from build123d import *

# Parameters (mm, degrees)
F0_R     = 4
F0_W     = 4
F0_H     = 4
F1_DEPTH = 10
F2_W     = 4.25
F2_H     = 4.25
F3_DEPTH = 7
F4_DEPTH = 6


with BuildPart() as f1:
    # F0 (on Top) → F1 (new body)
    with BuildSketch(Plane.XY):
        Circle(F0_R)
        Rectangle(F0_W, F0_H, mode=Mode.SUBTRACT)
        Rectangle(F0_W, F0_H)
    extrude(amount=F1_DEPTH)

    # F2 (on face) → F3 (cut)
    with BuildSketch(Plane.XY.offset(10)):
        Rectangle(F2_W, F2_H)
    extrude(amount=-F3_DEPTH, mode=Mode.SUBTRACT)

    # F0 (on Top) → F4 (join)
    with BuildSketch(Plane.XY):
        Rectangle(F0_W, F0_H)
    extrude(amount=-F4_DEPTH)


solid = f1.part
The listing builds one solid part. Answer for the finished solid, in the listing's coordinates (mm). A direction names the side the tool comes from. Round coordinates to 2 decimals unless told otherwise and drop trailing zeros. Order: outer loops, then holes, each group sorted by start corner. A loop starts at its lowest first (then second) coordinate and runs counter-clockwise, first axis right, second up. Notation, with made-up numbers: M 38.5,4 L 47.5,4 A14 cw 47.5,22 Z; hole C -1,23 d2. An arc over 180 degrees is marked long. Answer in a Markdown table with one row per item. Add a question column.
1) Flat-ended cylindrical pins translate along their axes: pin 1 Ø1 at (x, y) = (0.5, -1) entering from +Z; pin 2 Ø3 at (x, z) = (-1, -3.5) entering from +Y; pin 3 Ø1 at (x, z) = (-2.5, 3.5) entering from +Y. Find the tip coordinate at first contact, or state that the pin passes through.
2) Which of the six approach directions +Z, -Z, +X, -X, +Y, -Y give full straight-line access (tool end or side, diameter ignored) to faces 4 (the face through (0, 0, -6)), 5 (the face through (0, -2, -3)), 6 (the face through (0, 2.125, 7)), 7 (the face through (-2, 0, -3)), 8 (the face through (0, 2, -3))?
3) Consider line 1 along Z through (x, y) = (-3.25, 2); line 2 along X through (y, z) = (1.5, -4); line 3 along X through (y, z) = (0.75, 4) (3 decimals). Determine where each line is inside the solid, lowest interval first. Write a range as from..to.
4) The part is cut by section C-C on z = 7. Determine the outline of the cut face in (x, y) (3 decimals).
5) Determine the mould class of faces 1 (the face through (-0.867, -3.905, 4.93)), 2 (the face through (2.125, 0, 7)), 3 (the face through (2, 0, -3)) for opening direction Y: pulls with the +Y half, pulls with the -Y half, needs draft (parallel to the pull), parting line crosses it, or undercut.
6) The part is cut by section A-A on x = 0. Determine the outline of the cut face in (y, z) (3 decimals).
7) The part is cut by section D-D on z = 2. Determine the outline of the cut face in (x, y).
Findings below:
| question | item | result |
|---|---|---|
| 1 | pin 1 | stops at z = 3 |
| 1 | pin 2 | stops at y = 2 |
| 1 | pin 3 | stops at y = 3.46 |
| 2 | face 4 | -Z, +X, -X, +Y, -Y |
| 2 | face 5 | -Z, +X, -X, -Y |
| 2 | face 6 | +Z |
| 2 | face 7 | -Z, -X, +Y, -Y |
| 2 | face 8 | -Z, +X, -X, +Y |
| 3 | line 1 | z = 0..10 |
| 3 | line 2 | x = -2..2 |
| 3 | line 3 | x = -3.929..-2.125, 2.125..3.929 |
| 4 | outline | C 0,0 d8; hole M -2.125,-2.125 L 2.125,-2.125 L 2.125,2.125 L -2.125,2.125 Z |
| 5 | face 1 | parting line crosses it |
| 5 | face 2 | undercut |
| 5 | face 3 | needs draft |
| 6 | outline | M -4,0 L -2,0 L -2,-6 L 2,-6 L 2,0 L 4,0 L 4,10 L 2.125,10 L 2.125,3 L -2.125,3 L -2.125,10 L -4,10 Z |
| 7 | outline | C 0,0 d8 |
